Read the model definition and answer for the solid it produces. Units are mm, in the model's axes. Give positions to 0.01 mm unless a question says otherwise; leave off trailing zeros. Loops run counter-clockwise (first coordinate to the right, second up) from the corner with the lowest first, then second, coordinate; pieces in that order, holes last. Notation, with made-up numbers: (29, -32.5) -> (40, -32.5) arc R37 cw to (40, 6.5) -> close; hole circle Ø9 at (-2.75, 60.5). An arc over 180 degrees is marked (long way). Return JSON: item names as keys, results as strings. Group by question number.
from build123d import *

# Parameters (mm, degrees)
F0_R     = 50
F1_DEPTH = 100
F2_T     = -25
F3_R     = 1


with BuildPart() as f1:
    # F0 (on Top) → F1 (new body)
    with BuildSketch(Plane.XY):
        Circle(F0_R)
    extrude(amount=F1_DEPTH)

    # F2
    f2_openings = [f1.faces().sort_by_distance(p)[0] for p in [
        (0, 0, 100),
        (0, 0, 0),
    ]]
    offset(amount=F2_T, openings=f2_openings)

    # F3
    f3_edges = [f1.edges().sort_by_distance(p)[0] for p in [
        (-50, 0, 100),
        (-25, 0, 100),
        (-50, 0, 0),
        (-25, 0, 0),
    ]]
    fillet(f3_edges, radius=F3_R)


solid = f1.part
1. Section C-C on z = 28 is taken. Determine the outline of the cut face in (x, y).
2. Section A-A on x = 0 is taken. Determine the outline of the cut face in (y, z), then the cut area to 3 significant figures.
3. Straight lines are drawn through the part: line 1 (X direction, y = 1, z = 92); line 2 (Y direction, x = 0, z = 62); line 3 (Y direction, x = -13, z = 23). For each, find the intervals that lie inside material, in ascending order. Write a range as from..to.
4. Flat-ended cylindrical pins translate along their axes: pin 1 Ø8 at (y, z) = (-7, 52) entering from +X; pin 2 Ø5 at (x, z) = (-32.5, 70.5) entering from +Y; pin 3 Ø1.5 at (x, z) = (34, 57.5) entering from +Y. Find the tip coordinate at first contact, or state that the pin passes through.
5. Determine the mould class of faces 1 (the cylindrical face through (47.69, 15.02, 49.31)), 2 (the cylindrical face through (23.846, 7.509, 49.314)), 3 (the flat face through (21, -21, 100)) for opening direction X: pulls with the +X half, pulls with the -X half, needs draft (parallel to the pull), parting line crosses it, or undercut.
Completed:
{
 "1": {"outline": "circle Ø100 at (0, 0); hole circle Ø50 at (0, 0)"},
 "2": {"outline": "(-50, 1) arc R1 ccw to (-49, 0) -> (-26, 0) arc R1 ccw to (-25, 1) -> (-25, 99) arc R1 ccw to (-26, 100) -> (-49, 100) arc R1 ccw to (-50, 99) -> close; (25, 1) arc R1 ccw to (26, 0) -> (49, 0) arc R1 ccw to (50, 1) -> (50, 99) arc R1 ccw to (49, 100) -> (26, 100) arc R1 ccw to (25, 99) -> close", "area": "5,000 mm²"},
 "3": {"line 1": "x = -49.99..-24.98, 24.98..49.99", "line 2": "y = -50..-25, 25..50", "line 3": "y = -48.28..-21.35, 21.35..48.28"},
 "4": {"pin 1": "stops at x = 49.91", "pin 2": "stops at y = 40", "pin 3": "stops at y = 37.34"},
 "5": {"face 1": "parting line crosses it", "face 2": "undercut", "face 3": "needs draft"}
}
